Design review of the part built by this model. Coordinates are the model's own, in mm. A direction names the side the tool comes from. Give positions to 0.01 mm unless a question says otherwise; leave off trailing zeros. Loops run counter-clockwise (first coordinate to the right, second up) from the corner with the lowest first, then second, coordinate; pieces in that order, holes last. Notation, with made-up numbers: (-27, -10) -> (-16, -10) arc R23 ccw to (-16, 25) -> close; hole circle Ø10 at (49.25, 87). An arc over 180 degrees is marked (long way). Answer as CSV lines item,"result".
from build123d import *

# Parameters (mm, degrees)
SKETCH1_R               = 38.1
SKETCH1_R_2             = 6.35
BOSS_EXTRUDE1_DEPTH     = 36.5125
CUT_EXTRUDE2_DEPTH      = 66.0875
CUT_EXTRUDE2_DEPTH_BACK = 66.0875


with BuildPart() as part:
    # Sketch1 → Boss-Extrude1 (new body)
    with BuildSketch(Plane.XY):
        Circle(SKETCH1_R)
        Circle(SKETCH1_R_2, mode=Mode.SUBTRACT)
    extrude(amount=-BOSS_EXTRUDE1_DEPTH)

    # Sketch2 → Cut-Extrude2 (cut, two sides: drawn at the far end of the back side and taken through both)
    with BuildSketch(Plane(origin=(0, 0, 0), x_dir=(1, 0, 0), z_dir=(0, 1, 0)).offset(-CUT_EXTRUDE2_DEPTH_BACK)):
        Polygon((-38.1, 12.7), (-38.1, 0), (-25.4, 0), align=None)
        with BuildLine():
            Line((0, 0), (0, 4.7244))
            Line((0, 4.7244), (-24.339821656, 0.316401004))
            ThreePointArc((-24.339821656, 0.316401004), (-24.878689325, 0.187614988), (-25.4, 0))
            Line((-25.4, 0), (0, 0))
        make_face()
        with BuildLine():
            Line((24.339821656, 0.316401004), (0, 4.7244))
            Line((0, 4.7244), (0, 0))
            Line((0, 0), (25.4, 0))
            ThreePointArc((25.4, 0), (24.878689325, 0.187614988), (24.339821656, 0.316401004))
        make_face()
        Polygon((38.1, 12.7), (38.1, 0), (25.4, 0), align=None)
    extrude(amount=CUT_EXTRUDE2_DEPTH + CUT_EXTRUDE2_DEPTH_BACK, mode=Mode.SUBTRACT)


solid = part.part
Q1. We need section D-D, the plane y = 23. State the section outline as (x, z) points, and give its area (3 significant figures).
Filled sheet:
outline,"(-30.37, -36.51) -> (30.37, -36.51) -> (30.37, -4.97) -> (25.4, 0) arc R5 cw to (24.34, -0.32) -> (0, -4.72) -> (-24.34, -0.32) arc R5 cw to (-25.4, 0) -> (-30.37, -4.97) -> close"
area,"2,070 mm^2"
Q2. We need section B-B, the plane x = -5. State the section outline as (y, z) points, and give its area (3 significant figures).
Filled sheet:
outline,"(-37.77, -36.51) -> (-3.91, -36.51) -> (-3.91, -3.82) -> (-37.77, -3.82) -> close; (3.91, -36.51) -> (37.77, -36.51) -> (37.77, -3.82) -> (3.91, -3.82) -> close"
area,"2,210 mm^2"
Q3. We need section C-C, the plane z = -2.5. State the section outline as (x, y) points.
Filled sheet:
outline,"(-27.9, -25.95) arc R38.1 ccw to (-12.28, -36.07) -> (-12.28, 36.07) arc R38.1 ccw to (-27.9, 25.95) -> close; (12.28, -36.07) arc R38.1 ccw to (27.9, -25.95) -> (27.9, 25.95) arc R38.1 ccw to (12.28, 36.07) -> close"
Q4. To check wall thickness, follow probe 1 along Y at (x, z) = (0, -20); probe 2 along Y at (x, z) = (1.5, -22.5). State the ranges of each line that lie inside material, in increasing order. Write a range as from..to.
Filled sheet:
probe 1,"y = -38.1..-6.35, 6.35..38.1"
probe 2,"y = -38.07..-6.17, 6.17..38.07"
Q5. For faces 1 (the cylindrical face through (17.58, -33.8, -22.06)), 2 (the flat face through (12.34, -0.53, -2.49)), list the 3-axis set-ups (+Z, -Z, +X, -X, +Y, -Y) from which the entire face can be reached by the end or side of a thin tool; tool diameter is ignored.
Filled sheet:
face 1,"+Z, -Z"
face 2,"+Z, +Y, -Y"
Q6. Clearance check with flat-ended pins moving along their axes: pin 1 Ø8 at (x, z) = (25.5, -22) entering from -Y; pin 2 Ø2 at (x, z) = (19, -6) entering from -Y; pin 3 Ø1.5 at (x, z) = (9, -27) entering from -Y. State where each tip first meets the part, or that it passes through.
Filled sheet:
pin 1,"stops at y = -31.45"
pin 2,"stops at y = -33.58"
pin 3,"stops at y = -37.2"
Q7. We need section A-A, the plane y = 0. State the section outline as (x, z) points.
Filled sheet:
outline,"(-38.1, -36.51) -> (-6.35, -36.51) -> (-6.35, -3.57) -> (-24.34, -0.32) arc R5 cw to (-25.4, 0) -> (-38.1, -12.7) -> close; (6.35, -36.51) -> (38.1, -36.51) -> (38.1, -12.7) -> (25.4, 0) arc R5 cw to (24.34, -0.32) -> (6.35, -3.57) -> close"
Q8. The part is to be moulded in two halves that separate along X. For faces 3 (the flat face through (-12, -0.53, -2.55)), 4 (the flat face through (30.2, -0.4, -4.8)), 5 (the cylindrical face through (-1.38, -6.2, -19.81)), 6 (the flat face through (8, 1, -36.512)), say which applies: pulls with the +X half, pulls with the -X half, needs draft (parallel to the pull), parting line crosses it, or undercut.
Filled sheet:
face 3,"undercut"
face 4,"pulls with the +X half"
face 5,"undercut"
face 6,"needs draft"
